Here's how the part is built. I have some questions about the finished solid (model axes, mm). A direction names the side the tool comes from. Coordinates: 2 decimals unless noted, no trailing zeros. Order: outer loops, then holes, each group sorted by start corner. A loop starts at its lowest first (then second) coordinate and runs counter-clockwise, first axis right, second up.
```python
from build123d import *

# Parameters (mm, degrees)
BOSS_EXTRUDE1_DEPTH = 106
SKETCH3_R           = 1.7
BOSS_EXTRUDE2_DEPTH = 3.75
FILLET1_R           = 2.5


with BuildPart() as part:
    # Sketch2 → Boss-Extrude1 (new body)
    with BuildSketch(Plane.XY):
        with BuildLine():
            Line((2.75, 11.2), (2.75, 15))
            Line((2.75, 15), (-4.75, 15))
            Line((-4.75, 15), (-4.75, 0))
            Line((-4.75, 0), (2.75, 0))
            Line((2.75, 0), (2.75, 3.8))
            ThreePointArc((2.75, 3.8), (-0.95, 7.5), (2.75, 11.2))
        make_face()
    extrude(amount=-BOSS_EXTRUDE1_DEPTH)

    # Sketch3 → Boss-Extrude2 (add)
    # profile 1 of 2: a face of its own
    with BuildSketch(Plane.ZY.offset(-2.75)):
        with BuildLine():
            Line((-103.5, -10), (-97.5, -10))
            ThreePointArc((-97.5, -10), (-95.732233047, -9.267766953), (-95, -7.5))
            Line((-95, -7.5), (-95, 0))
            Line((-95, 0), (-10, 0))
            Line((-10, 0), (-10, -7.5))
            ThreePointArc((-10, -7.5), (-9.267766953, -9.267766953), (-7.5, -10))
            Line((-7.5, -10), (-2.5, -10))
            ThreePointArc((-2.5, -10), (-0.732233047, -9.267766953), (0, -7.5))
            Line((0, -7.5), (0, 3.8))
            Line((0, 3.8), (-106, 3.8))
            Line((-106, 3.8), (-106, -7.5))
            ThreePointArc((-106, -7.5), (-105.267766953, -9.267766953), (-103.5, -10))
        make_face()
        with Locations((-5, -5)):
            Circle(SKETCH3_R, mode=Mode.SUBTRACT)
        with Locations((-100, -5)):
            Circle(SKETCH3_R, mode=Mode.SUBTRACT)
    # profile 2 of 2: a face of its own
    with BuildSketch(Plane.ZY.offset(-2.75)):
        with BuildLine():
            Line((-106, 11.2), (0, 11.2))
            Line((0, 11.2), (0, 22.5))
            ThreePointArc((0, 22.5), (-0.732233047, 24.267766953), (-2.5, 25))
            Line((-2.5, 25), (-7.5, 25))
            ThreePointArc((-7.5, 25), (-9.267766953, 24.267766953), (-10, 22.5))
            Line((-10, 22.5), (-10, 15))
            Line((-10, 15), (-95, 15))
            Line((-95, 15), (-95, 22.5))
            ThreePointArc((-95, 22.5), (-95.732233047, 24.267766953), (-97.5, 25))
            Line((-97.5, 25), (-103.5, 25))
            ThreePointArc((-103.5, 25), (-105.267766953, 24.267766953), (-106, 22.5))
            Line((-106, 22.5), (-106, 11.2))
        make_face()
        with Locations((-5, 20)):
            Circle(SKETCH3_R, mode=Mode.SUBTRACT)
        with Locations((-100, 20)):
            Circle(SKETCH3_R, mode=Mode.SUBTRACT)
    extrude(amount=BOSS_EXTRUDE2_DEPTH)

    # Fillet1
    fillet1_edges = [part.edges().sort_by_distance(p)[0] for p in [
        (-4.75, 0, -53),
        (-4.75, 15, -53),
    ]]
    fillet(fillet1_edges, radius=FILLET1_R)


solid = part.part
```
Q1. If we section it at D-D on z = -37: Write out the boundary of the cut face in (x, y), then the cut area to 3 significant figures.
Q2. If we section it at C-C on x = 0: Write out the boundary of the cut face in (y, z), then the cut area to 3 significant figures.
Q3. For faces 4 (the flat face through (1, 19, -95)), 5 (the flat face through (-1, -5, -102)), 6 (the flat face through (1, -4, -10)), 7 (the flat face through (-1, 20, -102)), which set-ups out of +Z, -Z, +X, -X, +Y, -Y let a thin tool reach every point of the face, with its end or its side?
Q4. I need wall thicknesses on L1, parallel to Y at x = 1.2, z = -100; L2, parallel to Z at x = 0, y = -4; L3, parallel to Y at x = 0.05, z = -5. Which ranges of each line are inside material? Lowest first, please.
Q5. If we section it at B-B on y = 20: Write out the boundary of the cut face in (x, z).
Q6. We'd pull the mould along Y, two halves only. Please class faces 1 (the cylindrical face through (-0.95, 7.42, -52.26)), 2 (the cylindrical face through (0.901, 24.248, -0.713)), 3 (the cylindrical face through (-3.998, 0.713, -53.742)): pulls with the +Y half, pulls with the -Y half, needs draft (parallel to the pull), parting line crosses it, or undercut.
Q7. Will these pins go through, and if not, where does the flat tip stop? pin 1 (1 mm diameter, centred on x = 1.5, z = -64, fed in from -Y); pin 2 (1.5 mm diameter, centred on y = 8.5, z = -87, fed in from +X); pin 3 (3 mm diameter, centred on y = 20, z = -100, fed in from -X); pin 4 (8 mm diameter, centred on y = -4.5, z = -101, fed in from -X).
Q8. If we section it at A-A on z = -5: Write out the boundary of the cut face in (x, y).
Reply:
1. outline: (-4.75, 2.5) arc R2.5 ccw to (-2.25, 0) - (2.75, 0) - (2.75, 3.8) arc R3.7 cw to (2.75, 11.2) - (2.75, 15) - (-2.25, 15) arc R2.5 ccw to (-4.75, 12.5) - close
1. area: 88.3 mm2
2. outline: (-10, -103.5) arc R2.5 ccw to (-7.5, -106) - (5.02, -106) - (5.02, 0) - (-7.5, 0) arc R2.5 ccw to (-10, -2.5) - (-10, -7.5) arc R2.5 ccw to (-7.5, -10) - (0, -10) - (0, -95) - (-7.5, -95) arc R2.5 ccw to (-10, -97.5) - close; (9.98, -106) - (22.5, -106) arc R2.5 ccw to (25, -103.5) - (25, -97.5) arc R2.5 ccw to (22.5, -95) - (15, -95) - (15, -10) - (22.5, -10) arc R2.5 ccw to (25, -7.5) - (25, -2.5) arc R2.5 ccw to (22.5, 0) - (9.98, 0) - close; hole circle Ø3.4 at (-5, -100); hole circle Ø3.4 at (-5, -5); hole circle Ø3.4 at (20, -100); hole circle Ø3.4 at (20, -5)
2. area: 1,440 mm2
3. face 4: +X, -X, +Y
3. face 5: +Z, -Z, -X, -Y
3. face 6: +X, -X, -Y
3. face 7: +Z, -Z, -X, +Y
4. L1: y = -10 to -6.7, -3.3 to 4.14, 10.86 to 18.3, 21.7 to 25
4. L2: z = -106 to -101.37, -98.63 to -95, -10 to -6.37, -3.63 to 0
4. L3: y = -10 to -6.7, -3.3 to 4.97, 10.03 to 18.3, 21.7 to 25
5. outline: (-1, -106) - (2.75, -106) - (2.75, -101.7) - (-1, -101.7) - close; (-1, -98.3) - (2.75, -98.3) - (2.75, -95) - (-1, -95) - close; (-1, -10) - (2.75, -10) - (2.75, -6.7) - (-1, -6.7) - close; (-1, -3.3) - (2.75, -3.3) - (2.75, 0) - (-1, 0) - close
6. face 1: undercut
6. face 2: pulls with the +Y half
6. face 3: pulls with the -Y half
7. pin 1: stops at y = 0
7. pin 2: stops at x = -0.51
7. pin 3: passes through
7. pin 4: stops at x = -1
8. outline: (-4.75, 2.5) arc R2.5 ccw to (-2.25, 0) - (-1, 0) - (-1, -3.3) - (2.75, -3.3) - (2.75, 3.8) arc R3.7 cw to (2.75, 11.2) - (2.75, 18.3) - (-1, 18.3) - (-1, 15) - (-2.25, 15) arc R2.5 ccw to (-4.75, 12.5) - close; (-1, -10) - (2.75, -10) - (2.75, -6.7) - (-1, -6.7) - close; (-1, 21.7) - (2.75, 21.7) - (2.75, 25) - (-1, 25) - close
